Check sheet for the drawn part. Datum: minimum x, y, z corner. Units: mm. Give positions to 0.01 mm unless a question says otherwise; leave off trailing zeros. Write each loop counter-clockwise with the first axis right and the second up, starting at its lowest first coordinate (ties: lowest second). Pieces come first, ordered by that corner, then holes. Notation, with made-up numbers: (-29.5, 5) - (-1.5, 5) arc R38 ccw to (-1.5, 44) - close; hole circle Ø6 at (-12, -39). An arc over 180 degrees is marked (long way). Use a Markdown table: item, result.
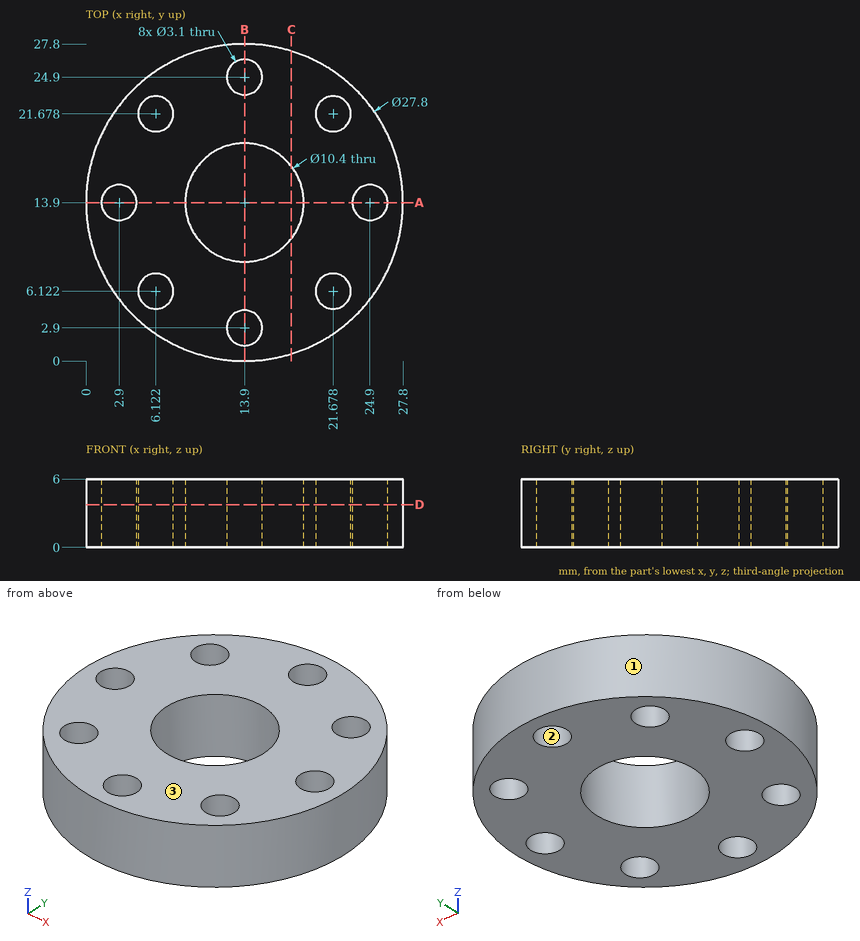
1) Section check C-C on x = 18. Record the boundary of the cut face in (y, z).
Working result:
| item | result |
|---|---|
| outline | (0.62, 0) - (10.7, 0) - (10.7, 6) - (0.62, 6) - close; (17.1, 0) - (27.18, 0) - (27.18, 6) - (17.1, 6) - close |
2) Section check A-A on y = 13.9. Record the boundary of the cut face in (x, z), then the cut area to 3 significant figures.
Working result:
| item | result |
|---|---|
| outline | (0, 0) - (1.35, 0) - (1.35, 6) - (0, 6) - close; (4.45, 0) - (8.7, 0) - (8.7, 6) - (4.45, 6) - close; (19.1, 0) - (23.35, 0) - (23.35, 6) - (19.1, 6) - close; (26.45, 0) - (27.8, 0) - (27.8, 6) - (26.45, 6) - close |
| area | 67.2 mm² |
3) Section check D-D on z = 3.75. Count the separate pieces of the cut face and the enclosed holes in it, then the cut area to 3 significant figures.
Working result:
| item | result |
|---|---|
| separate pieces | 1 |
| enclosed holes | 9 |
| area | 462 mm² |
4) Mould release check, pull along X, two halves, no side actions. Record for the marked faces 1, 2 and 3: pulls with the +X half, pulls with the -X half, needs draft (parallel to the pull), parting line crosses it, or undercut.
Working result:
| item | result |
|---|---|
| face 1 | parting line crosses it |
| face 2 | undercut |
| face 3 | needs draft |
5) Material ranges on L1, parallel to Y at x = 5.5, z = 3 (1 decimal); L2, parallel to X at y = 24, z = 0.65; L3, parallel to X at y = 25.75, z = 5.35 (1 decimal), recorded low to high. Write a range as from..to.
Working result:
| item | result |
|---|---|
| L1 | y = 2.8..4.7, 7.5..20.3, 23.1..25 |
| L2 | x = 4.35..12.64, 15.16..23.45 |
| L3 | x = 6.6..12.6, 15.2..21.2 |
